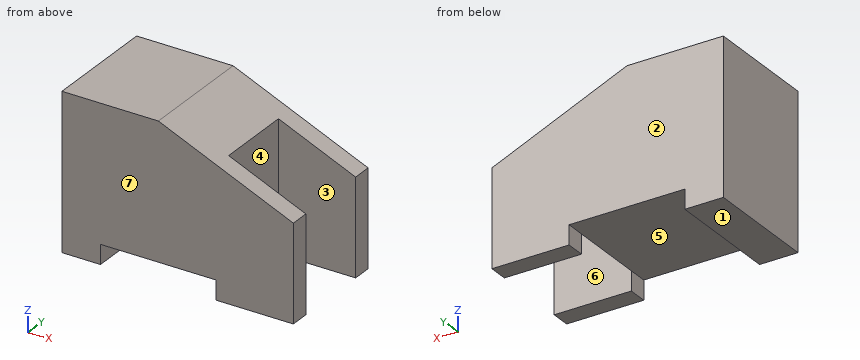
```python
from build123d import *

# Parameters (mm, degrees)
F1_DEPTH = 15
F2_DEPTH = 15
F3_W     = 10
F3_H     = 10
F4_DEPTH = 20.001
F5_DEPTH = 15.001


with BuildPart() as f1:
    # F0 (on Front) → F1 (new body)
    with BuildSketch(Plane.XZ):
        Polygon((0, 20), (0, 0), (5, 0), (5, 2.5), (20, 2.5), (20, 0), (30, 0), (30, 12.5), (12.5, 20), align=None)
    extrude(amount=-F1_DEPTH)

    # F0 (on Front) → F2 (join)
    with BuildSketch(Plane.XZ):
        Polygon((30, 20), (12.5, 20), (30, 12.5), align=None)
    extrude(amount=-F2_DEPTH)

    # F3 (on face) → F4 (cut, through all)
    with BuildSketch(Plane.XY.offset(20)):
        with Locations((25, 7.5)):
            Rectangle(F3_W, F3_H)
    extrude(amount=-F4_DEPTH, mode=Mode.SUBTRACT)

    # F0 (on Front) → F5 (cut, through all)
    with BuildSketch(Plane.XZ):
        Polygon((30, 20), (12.5, 20), (30, 12.5), align=None)
    extrude(amount=-F5_DEPTH, mode=Mode.SUBTRACT)


solid = f1.part
```
Geometry: final body of the model. Coordinates: model frame, mm. Face numbers are marked on the shaded views. A direction names the side the tool comes from. Give positions to 0.01 mm unless a question says otherwise; leave off trailing zeros. Write each loop counter-clockwise with the first axis right and the second up, starting at its lowest first coordinate (ties: lowest second). Pieces come first, ordered by that corner, then holes.
1. Section query D-D, the plane z = 18.25. Return loops of the section in (x, y).
2. Draft query along Y for the marked faces 1, 2, 3 and 4. Return one class per face: released by +Y, released by -Y, zero draft, split by the parting line, or undercut.
3. Reachability of the marked faces 5, 6 and 7 from +Z, -Z, +X, -X, +Y, -Y: full face, straight path, thin tool, end or side. Return the list, or none.
4. Line query: probe 1 along Y at (x, z) = (25, 13.75); probe 2 along X at (y, z) = (8, 12.25); probe 3 along Z at (x, y) = (7, 8.75). Output: solid intervals per line, ascending.
5. Pin query (flat end, axial travel): P1, Ø11, axis at x = 26.5, z = 5, coming from the -Y side; P2, Ø7.5, axis at x = 13, y = 11, coming from the -Z side; P3, Ø3, axis at y = 10, z = 1.5, coming from the +X side. Return the tip coordinate at first contact, or that it passes through.
6. Section query C-C, the plane x = 10.5. Return loops of the section in (y, z), then the cut area to 4 significant figures.
7. Section query A-A, the plane z = 9.25. Return loops of the section in (x, y).
8. Section query B-B, the plane y = 7.75. Return loops of the section in (x, z), then the cut area to 3 significant figures.
Computed:
1. outline: (0, 0) - (16.58, 0) - (16.58, 15) - (0, 15) - close
2. face 1: zero draft
2. face 2: released by +Y
2. face 3: undercut
2. face 4: undercut
3. face 5: -Z, +Y, -Y
3. face 6: +Z, -Z, +X
3. face 7: +Z, -Z, +X, -X, -Y
4. probe 1: y = 0 to 2.5, 12.5 to 15
4. probe 2: x = 0 to 20
4. probe 3: z = 2.5 to 20
5. P1: stops at y = 0
5. P2: stops at z = 2.5
5. P3: stops at x = 20
6. outline: (0, 2.5) - (15, 2.5) - (15, 20) - (0, 20) - close
6. area: 262.5 mm2
7. outline: (0, 0) - (30, 0) - (30, 2.5) - (20, 2.5) - (20, 12.5) - (30, 12.5) - (30, 15) - (0, 15) - close
8. outline: (0, 0) - (5, 0) - (5, 2.5) - (20, 2.5) - (20, 16.79) - (12.5, 20) - (0, 20) - close
8. area: 350 mm2
